Work out the finished part from the listing and answer in its coordinate system (mm). Face numbers are marked on the shaded views. A direction names the side the tool comes from. Round coordinates to 2 decimals unless told otherwise and drop trailing zeros. Write each loop counter-clockwise with the first axis right and the second up, starting at its lowest first coordinate (ties: lowest second). Pieces come first, ordered by that corner, then holes. Notation, with made-up numbers: (44, -8) - (53, -8) arc R17 cw to (53, 14) - close; hole circle Ø9 at (84, 35.5). An arc over 180 degrees is marked (long way). Answer as a JSON object with one key per item and string values.
```python
from build123d import *

# Parameters (mm, degrees)
F1_DEPTH       = 50
F2_D           = 8
F2_CBORE_D     = 9.75
F2_CBORE_DEPTH = 5
F3_D           = 15
F4_D           = 8.8
F4_CSINK_D     = 17.92
F4_CSINK_ANGLE = 90
F5_D           = 3.3
F6_SIZE2       = 2
F6_SIZE        = 2


with BuildPart() as f1:
    # F0 (on Top) → F1 (new body)
    with BuildSketch(Plane.XY):
        Polygon((-40, -40), (40, -40), (40, 40), (-40, 40), (-40, 12), (-17.0964375138, 12), (-17.0964375138, 0), (-40, 0), align=None)
    extrude(amount=F1_DEPTH)

    # F2 (through all)
    with Locations(Plane(origin=(0, 0, 0), x_dir=(1, 0, 0), z_dir=(0, 0, -1))):
        with Locations((-20, -20)):
            CounterBoreHole(F2_D / 2, F2_CBORE_D / 2, F2_CBORE_DEPTH)

    # F3 (through all)
    with Locations(Plane(origin=(0, 0, 0), x_dir=(1, 0, 0), z_dir=(0, 0, -1))):
        with Locations((20, -20)):
            Hole(F3_D / 2)

    # F4 (through all)
    with Locations(Plane(origin=(0, 0, 0), x_dir=(1, 0, 0), z_dir=(0, 0, -1))):
        with Locations((-20, 20)):
            CounterSinkHole(F4_D / 2, F4_CSINK_D / 2, counter_sink_angle=F4_CSINK_ANGLE)

    # F5 (through all)
    with Locations(Plane(origin=(0, 0, 0), x_dir=(1, 0, 0), z_dir=(0, 0, -1))):
        with Locations((20, 20)):
            Hole(F5_D / 2)

    # F6
    f6_edges = [f1.edges().sort_by_distance(p)[0] for p in [
        (-40, 40, 25),
        (-40, -20, 50),
        (-40, 26, 50),
        (-40, -40, 25),
        (-40, -20, 0),
        (-40, 26, 0),
        (0, 40, 0),
        (0, -40, 0),
        (40, 0, 0),
        (40, 0, 50),
        (0, 40, 50),
        (0, -40, 50),
        (40, -40, 25),
    ]]
    chamfer(f6_edges, length=F6_SIZE, length2=F6_SIZE2)


solid = f1.part
```
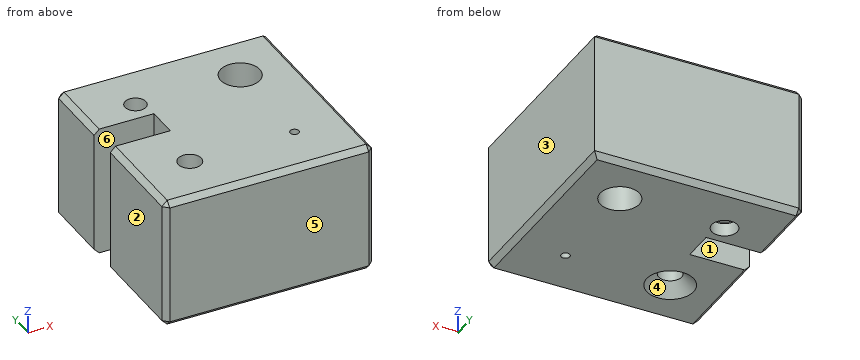
Item 1: A cutting plane is placed at A-A (y = 20). Write down the section's boundary in (x, z) (3 decimals), and give its area (3 significant figures).
Results found:
{"outline": "(-40, 2) - (-38, 0) - (-24.875, 0) - (-24.875, 5) - (-24, 5) - (-24, 50) - (-38, 50) - (-40, 48) - close; (-16, 5) - (-15.125, 5) - (-15.125, 0) - (12.5, 0) - (12.5, 50) - (-16, 50) - close; (27.5, 0) - (38, 0) - (40, 2) - (40, 48) - (38, 50) - (27.5, 50) - close", "area": "2,830 mm²"}
Item 2: Consider line 1 along Y through (x, z) = (20, 19); line 2 along X through (y, z) = (-20, 28); line 3 along Y through (x, z) = (-20, 29). Determine where each line is inside the solid, lowest interval first.
Results found:
{"line 1": "-40 to -21.65, -18.35 to 12.5, 27.5 to 40", "line 2": "-40 to -24.4, -15.6 to 18.35, 21.65 to 40", "line 3": "-40 to -24.4, -15.6 to 0, 12 to 16, 24 to 40"}
Item 3: A cutting plane is placed at D-D (x = 20). Write down the section's boundary in (y, z), and give its area (3 significant figures).
Results found:
{"outline": "(-40, 2) - (-38, 0) - (-21.65, 0) - (-21.65, 50) - (-38, 50) - (-40, 48) - close; (-18.35, 0) - (12.5, 0) - (12.5, 50) - (-18.35, 50) - close; (27.5, 0) - (38, 0) - (40, 2) - (40, 48) - (38, 50) - (27.5, 50) - close", "area": "3,080 mm²"}
Item 4: Determine the mould class of the marked faces 3, 4, 5 and 6 for opening direction Y: pulls with the +Y half, pulls with the -Y half, needs draft (parallel to the pull), parting line crosses it, or undercut.
Results found:
{"face 3": "needs draft", "face 4": "undercut", "face 5": "pulls with the -Y half", "face 6": "undercut"}
Item 5: Each of these flat-tipped pins is pushed along its axis until it touches: P1, Ø5, axis at x = -20, y = 20, coming from the -Z side; P2, Ø4, axis at y = 5, z = 44, coming from the -X side. Where does it stop, or does it pass through?
Results found:
{"P1": "through", "P2": "x = -17.1"}
Item 6: A cutting plane is placed at C-C (x = -20). Write down the section's boundary in (y, z) (3 decimals).
Results found:
{"outline": "(-40, 2) - (-38, 0) - (-28.96, 0) - (-24.4, 4.56) - (-24.4, 50) - (-38, 50) - (-40, 48) - close; (-15.6, 4.56) - (-11.04, 0) - (0, 0) - (0, 50) - (-15.6, 50) - close; (12, 0) - (15.125, 0) - (15.125, 5) - (16, 5) - (16, 50) - (12, 50) - close; (24, 5) - (24.875, 5) - (24.875, 0) - (38, 0) - (40, 2) - (40, 48) - (38, 50) - (24, 50) - close"}
Item 7: A cutting plane is placed at B-B (z = 30.5). Write down the section's boundary in (x, y).
Results found:
{"outline": "(-40, -38) - (-38, -40) - (38, -40) - (40, -38) - (40, 40) - (-38, 40) - (-40, 38) - (-40, 12) - (-17.1, 12) - (-17.1, 0) - (-40, 0) - close; hole circle Ø8.8 at (-20, -20); hole circle Ø8 at (-20, 20); hole circle Ø15 at (20, 20); hole circle Ø3.3 at (20, -20)"}
Item 8: For the marked faces 1 and 2, determine the directions among +Z, -Z, +X, -X, +Y, -Y from which every point of the face is accessible in a straight line to the end or side of a thin tool.
Results found:
{"face 1": "+Z, -Z, -X", "face 2": "+Z, -Z, -X, +Y, -Y"}
